Build history of the part. All positions in model axes, mm. Face numbers are marked on the shaded views. A direction names the side the tool comes from. Round coordinates to 2 decimals unless told otherwise and drop trailing zeros. Loops run counter-clockwise (first coordinate to the right, second up) from the corner with the lowest first, then second, coordinate; pieces in that order, holes last.
from build123d import *

# Parameters (mm, degrees)
SKETCH1_W           = 31.1
SKETCH1_H           = 26.1
BOSS_EXTRUDE1_DEPTH = 0.8
SKETCH2_W           = 20.3
SKETCH2_H           = 2.5
BOSS_EXTRUDE2_DEPTH = 2.5
SKETCH3_W           = 19
SKETCH3_H           = 0.6
BOSS_EXTRUDE3_DEPTH = 6.1
CHAMFER1_SIZE       = 0.2
SKETCH4_W           = 5.2
SKETCH4_H           = 3.6
BOSS_EXTRUDE4_DEPTH = 1
SKETCH5_W           = 0.2
SKETCH5_H           = 6
SKETCH5_W_2         = 3
SKETCH5_H_2         = 0.2
CUT_EXTRUDE1_DEPTH  = 0.1
SKETCH6_R           = 1.5
CUT_EXTRUDE2_DEPTH  = 23.718824794


with BuildPart() as part:
    # Sketch1 → Boss-Extrude1 (new, symmetric)
    with BuildSketch(Plane.XY):
        Rectangle(SKETCH1_W, SKETCH1_H)
    extrude(amount=BOSS_EXTRUDE1_DEPTH, both=True)

    # Sketch2 → Boss-Extrude2 (add)
    with BuildSketch(Plane(origin=(0, 0, -0.8), x_dir=(-1, 0, 0), z_dir=(0, 0, -1))):
        with Locations((0, -10.8)):
            Rectangle(SKETCH2_W, SKETCH2_H)
        with Locations((0, 10.8)):
            Rectangle(SKETCH2_W, SKETCH2_H)
    extrude(amount=BOSS_EXTRUDE2_DEPTH)

    # Sketch3 → Boss-Extrude3 (add)
    with BuildSketch(Plane(origin=(0, 0, -3.3), x_dir=(-1, 0, 0), z_dir=(0, 0, -1))):
        with Locations((0, 10.8)):
            Rectangle(SKETCH3_W, SKETCH3_H)
        with Locations((0, -10.8)):
            Rectangle(SKETCH3_W, SKETCH3_H)
    extrude(amount=BOSS_EXTRUDE3_DEPTH)

    # Chamfer1
    chamfer1_edges = [part.edges().sort_by_distance(p)[0] for p in [
        (9.5, 10.8, -9.4),
        (0, 10.5, -9.4),
        (-9.5, 10.8, -9.4),
        (0, 11.1, -9.4),
        (0, -11.1, -9.4),
        (-9.5, -10.8, -9.4),
        (0, -10.5, -9.4),
        (9.5, -10.8, -9.4),
    ]]
    chamfer(chamfer1_edges, length=CHAMFER1_SIZE)

    # Sketch4 → Boss-Extrude4 (add)
    with BuildSketch(Plane.XY.offset(0.8)):
        Rectangle(SKETCH4_W, SKETCH4_H)
    extrude(amount=BOSS_EXTRUDE4_DEPTH)

    # Sketch5 → Cut-Extrude1 (cut)
    with BuildSketch(Plane.XY.offset(0.8)):
        with Locations((-10.25, 4.35)):
            Rectangle(SKETCH5_W, SKETCH5_H)
        with Locations((-8.15, 0.75)):
            Rectangle(SKETCH5_W_2, SKETCH5_H_2)
    extrude(amount=-CUT_EXTRUDE1_DEPTH, mode=Mode.SUBTRACT)

    # Sketch6 → Cut-Extrude2 (cut, through all)
    with BuildSketch(Plane.XY.offset(0.8)):
        with Locations((-13.05, 10.55)):
            Circle(SKETCH6_R)
        with Locations((13.05, 10.55)):
            Circle(SKETCH6_R)
    extrude(amount=-CUT_EXTRUDE2_DEPTH, mode=Mode.SUBTRACT)


solid = part.part
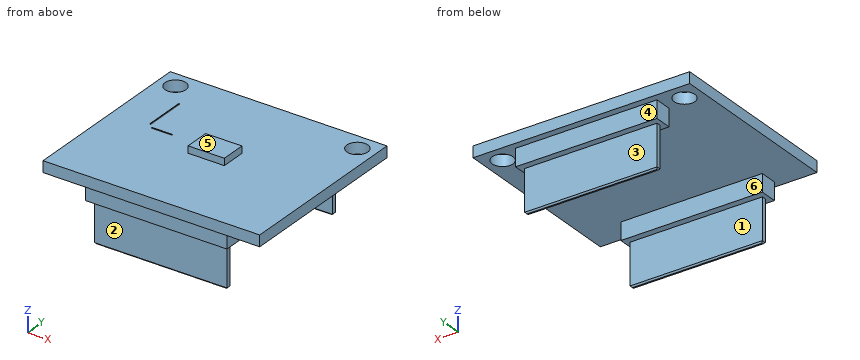
(1) Pull direction Y, two halves, no side cores. Call the marked faces 1, 2 and 3: +Y half, -Y half, draft (parallel to the pull), parting line (faces both ways), or undercut.
Responses:
face 1: undercut
face 2: -Y half
face 3: +Y half
(2) Slice it at D-D on x = 2. List the corners of the cut face in (y, z), plus the area to 3 significant figures.
Responses:
outline: (-13.05, -0.8) - (-12.05, -0.8) - (-12.05, -3.3) - (-11.1, -3.3) - (-11.1, -9.2) - (-10.9, -9.4) - (-10.7, -9.4) - (-10.5, -9.2) - (-10.5, -3.3) - (-9.55, -3.3) - (-9.55, -0.8) - (9.55, -0.8) - (9.55, -3.3) - (10.5, -3.3) - (10.5, -9.2) - (10.7, -9.4) - (10.9, -9.4) - (11.1, -9.2) - (11.1, -3.3) - (12.05, -3.3) - (12.05, -0.8) - (13.05, -0.8) - (13.05, 0.8) - (1.8, 0.8) - (1.8, 1.8) - (-1.8, 1.8) - (-1.8, 0.8) - (-13.05, 0.8) - close
area: 65.1 mm2
(3) Probe line 1 (Y direction, x = -13.05, z = 0.3); line 2 (Y direction, x = 0.5, z = -4.5); line 3 (X direction, y = -10, z = -1). List the from-to ranges inside material, lowest first.
Responses:
line 1: y = -13.05 to 9.05, 12.05 to 13.05
line 2: y = -11.1 to -10.5, 10.5 to 11.1
line 3: x = -10.15 to 10.15
(4) Which spindle directions (+Z, -Z, +X, -X, +Y, -Y) get a long thin tool onto all of the face, cutting with end or side? Do the marked faces 4, 5 and 6. Say none if no direction does.
Responses:
face 4: -Z, +X, -X, +Y
face 5: +Z, +X, -X, +Y, -Y
face 6: -Z, +X, -X
(5) Pin check, flat tips, straight feed: P1, Ø4, axis at x = 13.05, y = 10.55, coming from the +Z side; P2, Ø3, axis at x = -1.5, z = -5.5, coming from the +Y side; P3, Ø1, axis at x = 2, y = 1, coming from the -Z side; P4, Ø1.1, axis at y = 0.5, z = 1, coming from the -X side. Stop position of each tip, or through.
Responses:
P1: stops at z = 0.8
P2: stops at y = 11.1
P3: stops at z = -0.8
P4: stops at x = -15.55
(6) Slice it at A-A on x = -13.05. List the corners of the cut face in (y, z), plus the area to 3 significant figures.
Responses:
outline: (-13.05, -0.8) - (9.05, -0.8) - (9.05, 0.8) - (-13.05, 0.8) - close; (12.05, -0.8) - (13.05, -0.8) - (13.05, 0.8) - (12.05, 0.8) - close
area: 37.0 mm2
(7) Slice it at B-B on z = -1.75. List the corners of the cut face in (x, y), plus the area to 4 significant figures.
Responses:
outline: (-10.15, -12.05) - (10.15, -12.05) - (10.15, -9.55) - (-10.15, -9.55) - close; (-10.15, 9.55) - (10.15, 9.55) - (10.15, 12.05) - (-10.15, 12.05) - close
area: 101.5 mm2
(8) Slice it at C-C on y = 2.75. List the corners of the cut face in (x, z), plus the area to 3 significant figures.
Responses:
outline: (-15.55, -0.8) - (15.55, -0.8) - (15.55, 0.8) - (-10.15, 0.8) - (-10.15, 0.7) - (-10.35, 0.7) - (-10.35, 0.8) - (-15.55, 0.8) - close
area: 49.7 mm2
